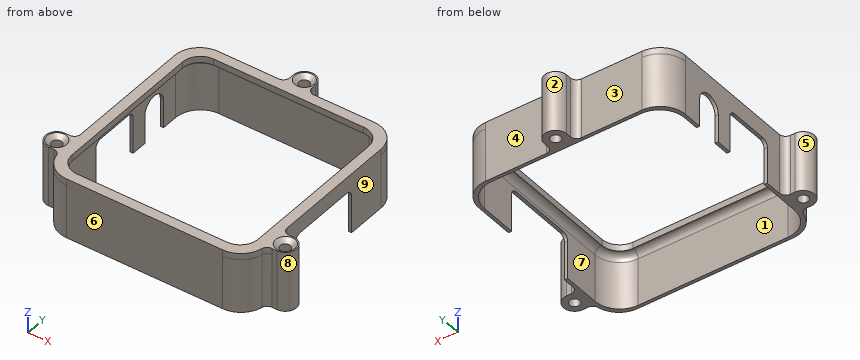
```python
from build123d import *

# Parameters (mm, degrees)
SKETCH1_W                                          = 103.175
SKETCH1_H                                          = 103.175
SKETCH1_W_2                                        = 100
SKETCH1_H_2                                        = 100
BOSS_EXTRUDE1_DEPTH                                = 26.9875
FILLET1_R                                          = 12.5
FILLET2_R                                          = 12.5
BOSS_EXTRUDE2_DEPTH                                = 3.175
CUT_EXTRUDE1_REACH                                 = 105.175
CUT_EXTRUDE2_REACH                                 = 105.175
CUT_EXTRUDE3_REACH                                 = 105.175
FILLET5_R                                          = 3.175
BOSS_EXTRUDE3_DEPTH                                = 30.1625
CSK_FOR_10_FLAT_HEAD_MACHINE_SCREW_100_D           = 5.1054
CSK_FOR_10_FLAT_HEAD_MACHINE_SCREW_100_DEPTH       = 30.1625
CSK_FOR_10_FLAT_HEAD_MACHINE_SCREW_100_CSINK_D     = 9.779
CSK_FOR_10_FLAT_HEAD_MACHINE_SCREW_100_CSINK_ANGLE = 100
FILLET4_R                                          = 3.175


with BuildPart() as part:
    # Sketch1 → Boss-Extrude1 (new body)
    with BuildSketch(Plane.XY):
        Rectangle(SKETCH1_W, SKETCH1_H)
        Rectangle(SKETCH1_W_2, SKETCH1_H_2, mode=Mode.SUBTRACT)
    extrude(amount=BOSS_EXTRUDE1_DEPTH)

    # Fillet1
    fillet1_edges = [part.edges().sort_by_distance(p)[0] for p in [
        (50, -50, 13.49375),
        (50, 50, 13.49375),
        (-50, 50, 13.49375),
        (-50, -50, 13.49375),
    ]]
    fillet(fillet1_edges, radius=FILLET1_R)

    # Fillet2
    fillet2_edges = [part.edges().sort_by_distance(p)[0] for p in [
        (51.5875, -51.5875, 13.49375),
        (-51.5875, -51.5875, 13.49375),
        (-51.5875, 51.5875, 13.49375),
        (51.5875, 51.5875, 13.49375),
    ]]
    fillet(fillet2_edges, radius=FILLET2_R)

    # Sketch2 → Boss-Extrude2 (add)
    with BuildSketch(Plane.XY.offset(26.9875)):
        with BuildLine():
            Line((-39.0875, -51.5875), (39.0875, -51.5875))
            ThreePointArc((39.0875, -51.5875), (47.926334765, -47.926334765), (51.5875, -39.0875))
            Line((51.5875, -39.0875), (51.5875, 39.0875))
            ThreePointArc((51.5875, 39.0875), (47.926334765, 47.926334765), (39.0875, 51.5875))
            Line((39.0875, 51.5875), (-39.0875, 51.5875))
            ThreePointArc((-39.0875, 51.5875), (-47.926334765, 47.926334765), (-51.5875, 39.0875))
            Line((-51.5875, 39.0875), (-51.5875, -39.0875))
            ThreePointArc((-51.5875, -39.0875), (-47.926334765, -47.926334765), (-39.0875, -51.5875))
        make_face()
        with BuildLine():
            Line((46.5, -37.5), (46.5, 37.5))
            ThreePointArc((46.5, 37.5), (43.863961031, 43.863961031), (37.5, 46.5))
            Line((37.5, 46.5), (-37.5, 46.5))
            ThreePointArc((-37.5, 46.5), (-43.863961031, 43.863961031), (-46.5, 37.5))
            Line((-46.5, 37.5), (-46.5, -37.5))
            ThreePointArc((-46.5, -37.5), (-43.863961031, -43.863961031), (-37.5, -46.5))
            Line((-37.5, -46.5), (37.5, -46.5))
            ThreePointArc((37.5, -46.5), (43.863961031, -43.863961031), (46.5, -37.5))
        make_face(mode=Mode.SUBTRACT)
    extrude(amount=BOSS_EXTRUDE2_DEPTH)

    # Sketch3 → Cut-Extrude1 (cut, up to next)
    with BuildSketch(Plane.ZY.offset(51.5875), mode=Mode.PRIVATE) as cut_extrude1_sk1:
        with BuildLine():
            Line((0, 29.3625), (13.97, 29.3625))
            ThreePointArc((13.97, 29.3625), (20.32, 23.0125), (13.97, 16.6625))
            Line((13.97, 16.6625), (0, 16.6625))
            ThreePointArc((0, 16.6625), (-6.35, 23.0125), (0, 29.3625))
        make_face()
    cut_extrude1_tool1 = extrude(cut_extrude1_sk1.sketch, amount=-CUT_EXTRUDE1_REACH, mode=Mode.PRIVATE) & part.part
    add(cut_extrude1_tool1.solids().sort_by_distance((-51.5875, 23.0125, 6.985))[0], mode=Mode.SUBTRACT)

    # Sketch5 → Cut-Extrude2 (cut, up to next)
    with BuildSketch(Plane.ZY.offset(51.5875), mode=Mode.PRIVATE) as cut_extrude2_sk1:
        Polygon((8.73125, -16.6625), (21.43125, -16.6625), (21.43125, 8.7375), (8.73125, 8.7375), (0, 8.7375), (0, -16.6625), align=None)
    cut_extrude2_tool1 = extrude(cut_extrude2_sk1.sketch, amount=-CUT_EXTRUDE2_REACH, mode=Mode.PRIVATE) & part.part
    add(cut_extrude2_tool1.solids().sort_by_distance((-51.5875, -3.9625, 10.715625))[0], mode=Mode.SUBTRACT)

    # Sketch6 → Cut-Extrude3 (cut, up to next)
    with BuildSketch(Plane(origin=(51.5875, 0, 0), x_dir=(0, 0, -1), z_dir=(1, 0, 0)), mode=Mode.PRIVATE) as cut_extrude3_sk1:
        Polygon((-3.175, -19.05), (-22.225, -19.05), (-22.225, 19.05), (-3.175, 19.05), (0, 19.05), (0, -19.05), align=None)
    cut_extrude3_tool1 = extrude(cut_extrude3_sk1.sketch, amount=-CUT_EXTRUDE3_REACH, mode=Mode.PRIVATE) & part.part
    add(cut_extrude3_tool1.solids().sort_by_distance((51.5875, 0, 11.1125))[0], mode=Mode.SUBTRACT)

    # Fillet5
    fillet5_edges = [part.edges().sort_by_distance(p)[0] for p in [
        (-50.79375, -16.6625, 21.43125),
        (-50.79375, 8.7375, 21.43125),
        (50.79375, 19.05, 22.225),
        (50.79375, -19.05, 22.225),
        (50, 0, 26.9875),
        (0, 50, 26.9875),
        (0, -50, 26.9875),
        (-50, 0, 26.9875),
        (46.338834765, 46.338834765, 26.9875),
        (46.338834765, -46.338834765, 26.9875),
        (-46.338834765, -46.338834765, 26.9875),
        (-46.338834765, 46.338834765, 26.9875),
    ]]
    fillet(fillet5_edges, radius=FILLET5_R)

    # Sketch7 → Boss-Extrude3 (add)
    with BuildSketch(Plane.XY.offset(30.1625)):
        with BuildLine():
            Line((57.14375, -27.975), (51.5875, -27.975))
            Line((51.5875, -27.975), (51.5875, -39.0875))
            Line((51.5875, -39.0875), (57.14375, -39.0875))
            ThreePointArc((57.14375, -39.0875), (62.7, -33.53125), (57.14375, -27.975))
        make_face()
        with BuildLine():
            Line((-51.5875, -39.0875), (-57.14375, -39.0875))
            ThreePointArc((-57.14375, -39.0875), (-62.7, -33.53125), (-57.14375, -27.975))
            Line((-57.14375, -27.975), (-51.5875, -27.975))
            Line((-51.5875, -27.975), (-51.5875, -39.0875))
        make_face()
        with BuildLine():
            Line((-5.55625, 51.5875), (5.55625, 51.5875))
            Line((5.55625, 51.5875), (5.55625, 57.14375))
            ThreePointArc((5.55625, 57.14375), (0, 62.7), (-5.55625, 57.14375))
            Line((-5.55625, 57.14375), (-5.55625, 51.5875))
        make_face()
    extrude(amount=-BOSS_EXTRUDE3_DEPTH)

    # CSK for #10 Flat Head Machine Screw (100)1
    with Locations(Plane(origin=(57.14375, -33.53125, 30.1625), x_dir=(1, 0, 0), z_dir=(0, 0, 1))):
        with Locations((0, 0), (-114.2875, 0), (-57.14375, 90.675)):
            CounterSinkHole(CSK_FOR_10_FLAT_HEAD_MACHINE_SCREW_100_D / 2, CSK_FOR_10_FLAT_HEAD_MACHINE_SCREW_100_CSINK_D / 2, depth=CSK_FOR_10_FLAT_HEAD_MACHINE_SCREW_100_DEPTH, counter_sink_angle=CSK_FOR_10_FLAT_HEAD_MACHINE_SCREW_100_CSINK_ANGLE)

    # Fillet4
    fillet4_edges = [part.edges().sort_by_distance(p)[0] for p in [
        (51.5875, -27.975, 15.08125),
        (-51.5875, -27.975, 15.08125),
        (5.55625, 51.5875, 15.08125),
        (-5.55625, 51.5875, 15.08125),
        (51.5875, -39.0875, 15.08125),
        (-51.5875, -39.0875, 15.08125),
    ]]
    fillet(fillet4_edges, radius=FILLET4_R)


solid = part.part
```
Build history of the part. All positions in model axes, mm. Face numbers are marked on the shaded views. A direction names the side the tool comes from. Round coordinates to 2 decimals unless told otherwise and drop trailing zeros. Answer in a Markdown table with one row per item.
1) Band-saw the part on C-C on z = 8. Give the number of separate pieces and of enclosed holes in the cut face, and give its area (3 significant figures).
Values:
| item | result |
|---|---|
| separate pieces | 3 |
| enclosed holes | 3 |
| area | 805 mm2 |
2) Mould opens along Y. For the marked faces 6, 7, 8 and 9 say: released by +Y, released by -Y, zero draft, split by the parting line, or undercut.
Values:
| item | result |
|---|---|
| face 6 | released by -Y |
| face 7 | undercut |
| face 8 | split by the parting line |
| face 9 | zero draft |
3) Which spindle directions (+Z, -Z, +X, -X, +Y, -Y) get a long thin tool onto all of the face, cutting with end or side? Do the marked faces 1, 2, 3, 4 and 5. Say none if no direction does.
Values:
| item | result |
|---|---|
| face 1 | -Z |
| face 2 | +Z, -Z, +Y |
| face 3 | +Z, -Z, -X, +Y |
| face 4 | +Z, -Z, +X, +Y |
| face 5 | +Z, -Z, -X |
4) Wall check: L1, parallel to Y at x = 0, z = 21.5; L2, parallel to X at y = -20, z = 1. Give the ranges that are in metal, low to high.
Values:
| item | result |
|---|---|
| L1 | -51.59 to -50, 50 to 54.59, 59.7 to 62.7 |
| L2 | -51.59 to -50, 50 to 51.59 |
5) Pin check, flat tips, straight feed: P1, Ø1, axis at y = -1, z = 28.5, coming from the -X side; P2, Ø1.3, axis at x = 51, y = 7.5, coming from the -Z side (3 decimals); P3, Ø9, axis at x = 22, z = 8, coming from the +Y side; P4, Ø6, axis at x = 40.5, z = 14, coming from the -Y side. Stop position of each tip, or through.
Values:
| item | result |
|---|---|
| P1 | x = -51.59 |
| P2 | z = 22.225 |
| P3 | y = 51.59 |
| P4 | y = -51.59 |
